```python
from build123d import *

# Parameters (mm, degrees)
SKETCH1_W            = 18.542
SKETCH1_H            = 17.78
BOSS_EXTRUDE4_DEPTH  = 1.905
SKETCH4_W            = 18.542
SKETCH4_H            = 17.78
BOSS_EXTRUDE5_DEPTH  = 1.905
BOSS_EXTRUDE6_DEPTH  = 18.542
SKETCH7_W            = 8.89
SKETCH7_H            = 10.16
BOSS_EXTRUDE7_DEPTH  = 1.905
SKETCH8_W            = 8.89
SKETCH8_H            = 10.16
BOSS_EXTRUDE8_DEPTH  = 1.905
SKETCH12_W           = 12.7
SKETCH12_H           = 12.7
BOSS_EXTRUDE11_DEPTH = 2.286
CUT_EXTRUDE2_DEPTH   = 22.721455683


with BuildPart() as part:
    # Sketch1 → Boss-Extrude4 (new body)
    with BuildSketch(Plane.XY):
        Rectangle(SKETCH1_W, SKETCH1_H)
    extrude(amount=-BOSS_EXTRUDE4_DEPTH)



with BuildPart() as body_2:
    # Sketch4 → Boss-Extrude5 (new body)
    with BuildSketch(Plane.XY.offset(-12.7)):
        Rectangle(SKETCH4_W, SKETCH4_H)
    extrude(amount=BOSS_EXTRUDE5_DEPTH)


with BuildPart() as part_1:
    add(part.part)

    add(body_2.part)  # Boss-Extrude6 merges body 2
    # Sketch6 → Boss-Extrude6 (add)
    with BuildSketch(Plane.ZY.offset(9.271)):
        with BuildLine():
            Line((-12.7, 8.89), (-10.795, 8.89))
            ThreePointArc((-10.795, 8.89), (-6.35, 13.335), (-1.905, 8.89))
            Line((-1.905, 8.89), (0, 8.89))
            ThreePointArc((0, 8.89), (-6.35, 15.24), (-12.7, 8.89))
        make_face()
    extrude(amount=-BOSS_EXTRUDE6_DEPTH)

    # Sketch7 → Boss-Extrude7 (add)
    with BuildSketch(Plane.ZY.offset(9.271)):
        with Locations((-6.35, -3.81)):
            Rectangle(SKETCH7_W, SKETCH7_H)
    extrude(amount=-BOSS_EXTRUDE7_DEPTH)

    # Sketch8 → Boss-Extrude8 (add)
    with BuildSketch(Plane(origin=(9.271, 0, 0), x_dir=(0, 0, -1), z_dir=(1, 0, 0))):
        with Locations((6.35, -3.81)):
            Rectangle(SKETCH8_W, SKETCH8_H)
    extrude(amount=-BOSS_EXTRUDE8_DEPTH)

    # Sketch12 → Boss-Extrude11 (add)
    with BuildSketch(Plane(origin=(0, 0, -12.7), x_dir=(-1, 0, 0), z_dir=(0, 0, -1))):
        with Locations((0, -2.54)):
            Rectangle(SKETCH12_W, SKETCH12_H)
    extrude(amount=BOSS_EXTRUDE11_DEPTH)

    # Sketch13 → Cut-Extrude2 (cut, through all)
    with BuildSketch(Plane(origin=(0, 3.81, 0), x_dir=(1, 0, 0), z_dir=(0, 1, 0))):
        Polygon((-5.08, 12.7), (5.08, 12.7), (5.08, 14.478), (-5.08, 14.420748278), align=None)
    extrude(amount=-CUT_EXTRUDE2_DEPTH, mode=Mode.SUBTRACT)


solid = part_1.part
```
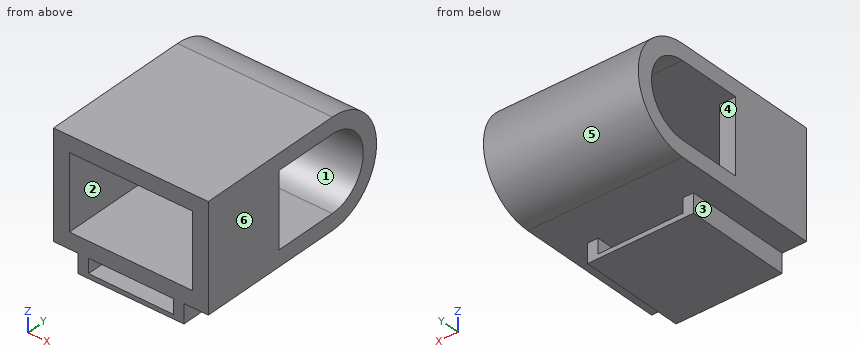
Can you work these out from the model? Positions are in its coordinate system, mm. Face numbers are marked on the shaded views. A direction names the side the tool comes from. Coordinates: 2 decimals unless noted, no trailing zeros. Loops run counter-clockwise (first coordinate to the right, second up) from the corner with the lowest first, then second, coordinate; pieces in that order, holes last.
Item 1: Please list where these lines run through material, in increasing order: L1, parallel to Z at x = -4, y = -6.25 (3 decimals); L2, parallel to X at y = -3, z = -8.25; L3, parallel to X at y = -1, z = -13.
Answers below:
L1: z = -14.986 to -14.427, -12.7 to -10.795, -1.905 to 0
L2: x = -9.27 to -7.37, 7.37 to 9.27
L3: x = -6.35 to -5.08, 5.08 to 6.35
Item 2: I'm going to push flat-ended pins straight in: pin 1 (6 mm diameter, centred on x = -1, y = 8.5, fed in from -Z); pin 2 (0.5 mm diameter, centred on y = -1.5, z = -13.5, fed in from -X); pin 3 (2 mm diameter, centred on x = 8, z = -8, fed in from +Y). Where does each tip first touch, or does it pass through?
Answers below:
pin 1: stops at z = -12.7
pin 2: stops at x = -6.35
pin 3: stops at y = 15.21
Item 3: If we mould it in two halves opening along Y, with no side actions, what happens to the marked faces 4, 5 and 6? For each: released by +Y, released by -Y, zero draft, split by the parting line, or undercut.
Answers below:
face 4: undercut
face 5: released by +Y
face 6: zero draft
Item 4: Suppose I cut it at D-D (z = -14). Please give me the cut outline in (x, y), then the cut area to 3 significant figures.
Answers below:
outline: (-6.35, -8.89) - (-5.08, -8.89) - (-5.08, 3.81) - (-6.35, 3.81) - close; (5.08, -8.89) - (6.35, -8.89) - (6.35, 3.81) - (5.08, 3.81) - close
area: 32.3 mm2
Item 5: Suppose I cut it at B-B (x = 3.25). Please give me the cut outline in (y, z) (3 decimals).
Answers below:
outline: (-8.89, -14.986) - (3.81, -14.986) - (3.81, -14.468) - (-8.89, -14.468) - close; (-8.89, -12.7) - (8.89, -12.7) arc R6.35 ccw to (8.89, 0) - (-8.89, 0) - (-8.89, -1.905) - (8.89, -1.905) arc R4.445 cw to (8.89, -10.795) - (-8.89, -10.795) - close
Item 6: Suppose I cut it at C-C (y = 13). Please give me the cut outline in (x, z), then the cut area to 3 significant figures.
Answers below:
outline: (-9.27, -11.19) - (9.27, -11.19) - (9.27, -8.04) - (-9.27, -8.04) - close; (-9.27, -4.66) - (9.27, -4.66) - (9.27, -1.51) - (-9.27, -1.51) - close
area: 117 mm2
Item 7: Suppose I cut it at A-A (z = -6.35). Please give me the cut outline in (x, y) (3 decimals).
Answers below:
outline: (-9.271, -8.89) - (-7.366, -8.89) - (-7.366, 1.27) - (-9.271, 1.27) - close; (-9.271, 13.335) - (9.271, 13.335) - (9.271, 15.24) - (-9.271, 15.24) - close; (7.366, -8.89) - (9.271, -8.89) - (9.271, 1.27) - (7.366, 1.27) - close
Item 8: Which directions (+Z, -Z, +X, -X, +Y, -Y) give clear straight access to the entire face, cutting with the end or side of a thin tool? Please do the marked faces 1, 2 and 3.
Answers below:
face 1: +X, -X
face 2: -Y
face 3: -Z, -X, +Y, -Y
